Here's how the part is built. I have some questions about the finished solid (model axes, mm). A direction names the side the tool comes from. Round coordinates to 2 decimals unless told otherwise and drop trailing zeros. Write each loop counter-clockwise with the first axis right and the second up, starting at its lowest first coordinate (ties: lowest second). Pieces come first, ordered by that corner, then holes. Notation, with made-up numbers: (48, 50) - (81, 50) arc R24 ccw to (81, 75) - close; hole circle Ø9 at (-30, 14). An arc over 180 degrees is marked (long way). One line per item, written item: value. Start each with the question number.
Item 1: Imagine slicing it at C-C, the plane x = -77.5. Please give me the cut outline in (y, z) (3 decimals).
Item 2: Imagine slicing it at B-B, the plane y = 69. Please give me the cut outline in (x, z) (3 decimals).
Item 3: Imagine slicing it at A-A, the plane z = 2.4. Count the separate pieces of the cut face and the enclosed holes in it, then the cut area to 3 significant figures.
Item 4: For P1, Ø1.5, axis at y = 17, z = 1.5, coming from the +X side, with a flat end and sliding along its axis, tell me the tip position at first contact or that it passes through.
Item 5: Thinking about a two-plate mould opening in Y: for faces 3 (the face through (-59, 17, 0)), 4 (the face through (-67.62, 108.19, 1.57)), 5 (the face through (-51.137, -4.439, 1.61)), 6 (the face through (-13.2, -21.2, 1.6)), which applies, released by +Y, released by -Y, zero draft, split by the parting line, or undercut?
Item 6: If I drill on line 1 (X direction, y = 32, z = 1.1); line 2 (X direction, y = 79, z = 3); line 3 (Y direction, x = -12, z = 2.9), over which ranges is the centre line in solid material (lowest first)?
Item 7: For faces 1 (the face through (-59, 17, 3.175)), 2 (the face through (-3.89, 77.18, 1.61)), which set-ups out of +Z, -Z, +X, -X, +Y, -Y let a thin tool reach every point of the face, with its end or its side?
```python
from build123d import *

# Parameters (mm, degrees)
F0_R     = 76.2
F1_DEPTH = 3.175
F3_DEPTH = 25.4
F4_DEPTH = 25.4


with BuildPart() as f1:
    # F0 (on Top) → F1 (new body)
    with BuildSketch(Plane.XY):
        with Locations((-57.6965734363, 32.640516758)):
            Circle(F0_R)
    extrude(amount=F1_DEPTH)

    # F2 (on face) → F3 (cut)
    with BuildSketch(Plane.XY.offset(3.175)):
        with BuildLine():
            ThreePointArc((-126.4787083378, 20.4733306254), (-111.1800565213, -12.2876429762), (-81.5505486037, -33.0101524596))
            Line((-81.5505486037, -33.0101524596), (-59.8651166333, 26.6722741018))
            ThreePointArc((-59.8651166333, 26.6722741018), (-62.5587082622, 28.5561386003), (-63.9494947909, 31.5344089277))
            Line((-63.9494947909, 31.5344089277), (-126.4787083378, 20.4733306254))
        make_face()
        with BuildLine():
            Line((-58.8026812665, 38.8934381127), (-69.8637595688, 101.4226516595))
            ThreePointArc((-69.8637595688, 101.4226516595), (-102.6247331704, 86.123999843), (-123.3472426538, 56.4944919254))
            Line((-123.3472426538, 56.4944919254), (-63.6648160924, 34.809059955))
            ThreePointArc((-63.6648160924, 34.809059955), (-61.7809515939, 37.5026515839), (-58.8026812665, 38.8934381127))
        make_face()
        with BuildLine():
            ThreePointArc((-45.5293873037, -36.1416181436), (-12.7684137021, -20.842966327), (7.9540957813, 8.7865415905))
            Line((7.9540957813, 8.7865415905), (-51.7283307801, 30.4719735609))
            ThreePointArc((-51.7283307801, 30.4719735609), (-53.6121952786, 27.7783819321), (-56.590465606, 26.3875954033))
            Line((-56.590465606, 26.3875954033), (-45.5293873037, -36.1416181436))
        make_face()
        with BuildLine():
            Line((-51.4436520816, 33.7466245882), (11.0855614653, 44.8077028905))
            ThreePointArc((11.0855614653, 44.8077028905), (-4.2130903513, 77.5686764921), (-33.8425982688, 98.2911859755))
            Line((-33.8425982688, 98.2911859755), (-55.5280302392, 38.6087594141))
            ThreePointArc((-55.5280302392, 38.6087594141), (-52.8344386104, 36.7248949156), (-51.4436520816, 33.7466245882))
        make_face()
    extrude(amount=-F3_DEPTH, mode=Mode.SUBTRACT)

    # F2 (on face) → F4 (cut)
    with BuildSketch(Plane.XY.offset(3.175)):
        with BuildLine():
            ThreePointArc((-57.4200464787, 31.0772864193), (-56.6754788968, 31.4249830515), (-56.2045127722, 32.0983809587))
            Line((-56.2045127722, 32.0983809587), (-57.6965734363, 32.640516758))
            Line((-57.6965734363, 32.640516758), (-57.4200464787, 31.0772864193))
        make_face()
        with BuildLine():
            ThreePointArc((-56.1090734363, 32.640516758), (-56.1151524909, 32.7793117279), (-56.1333430976, 32.9170437155))
            Line((-56.1333430976, 32.9170437155), (-57.6965734363, 32.640516758))
            Line((-57.6965734363, 32.640516758), (-56.2045127722, 32.0983809587))
            ThreePointArc((-56.2045127722, 32.0983809587), (-56.1331153214, 32.365280545), (-56.1090734363, 32.640516758))
        make_face()
        with BuildLine():
            Line((-57.6965734363, 32.640516758), (-56.1333430976, 32.9170437155))
            ThreePointArc((-56.1333430976, 32.9170437155), (-56.4810397298, 33.6616112974), (-57.154437637, 34.132577422))
            Line((-57.154437637, 34.132577422), (-57.6965734363, 32.640516758))
        make_face()
        with BuildLine():
            Line((-57.6965734363, 32.640516758), (-57.154437637, 34.132577422))
            ThreePointArc((-57.154437637, 34.132577422), (-57.5590841827, 34.2220517576), (-57.9731003938, 34.2037470966))
            Line((-57.9731003938, 34.2037470966), (-57.6965734363, 32.640516758))
        make_face()
        with BuildLine():
            Line((-59.1886341003, 33.1826525572), (-57.6965734363, 32.640516758))
            Line((-57.6965734363, 32.640516758), (-57.9731003938, 34.2037470966))
            ThreePointArc((-57.9731003938, 34.2037470966), (-58.7176679757, 33.8560504644), (-59.1886341003, 33.1826525572))
        make_face()
        with BuildLine():
            Line((-59.2598037749, 32.3639898004), (-57.6965734363, 32.640516758))
            Line((-57.6965734363, 32.640516758), (-59.1886341003, 33.1826525572))
            ThreePointArc((-59.1886341003, 33.1826525572), (-59.2781084359, 32.7780060115), (-59.2598037749, 32.3639898004))
        make_face()
        with BuildLine():
            Line((-58.2387092355, 31.1484560939), (-57.6965734363, 32.640516758))
            Line((-57.6965734363, 32.640516758), (-59.2598037749, 32.3639898004))
            ThreePointArc((-59.2598037749, 32.3639898004), (-58.9121071427, 31.6194222186), (-58.2387092355, 31.1484560939))
        make_face()
        with BuildLine():
            Line((-57.4200464787, 31.0772864193), (-57.6965734363, 32.640516758))
            Line((-57.6965734363, 32.640516758), (-58.2387092355, 31.1484560939))
            ThreePointArc((-58.2387092355, 31.1484560939), (-57.8340626898, 31.0589817583), (-57.4200464787, 31.0772864193))
        make_face()
    extrude(amount=-F4_DEPTH, mode=Mode.SUBTRACT)


solid = f1.part
```
Values follow:
1. outline: (-40.941, 0) - (-21.862, 0) - (-21.862, 3.175) - (-40.941, 3.175) - close; (29.137, 0) - (39.836, 0) - (39.836, 3.175) - (29.137, 3.175) - close; (99.624, 0) - (106.222, 0) - (106.222, 3.175) - (99.624, 3.175) - close
2. outline: (-124.662, 0) - (-117.337, 0) - (-117.337, 3.175) - (-124.662, 3.175) - close; (-64.128, 0) - (-44.485, 0) - (-44.485, 3.175) - (-64.128, 3.175) - close; (1.944, 0) - (9.269, 0) - (9.269, 3.175) - (1.944, 3.175) - close
3. separate pieces: 1
3. enclosed holes: 5
3. area: 8,100 mm^2
4. P1: stops at x = 17.03
5. face 3: zero draft
5. face 4: split by the parting line
5. face 5: undercut
5. face 6: undercut
6. line 1: x = -133.89 to -59.15, -56.24 to 18.5
6. line 2: x = -118.17 to -109.94, -65.9 to -40.85, -5.45 to 2.78
6. line 3: y = -28.34 to -20.19, 16.04 to 40.72, 85.47 to 93.62
7. face 1: +Z, +X, -X, +Y, -Y
7. face 2: +Z, -Z
